Geometry: final body of the model. Coordinates: model frame, mm. A direction names the side the tool comes from. Give positions to 0.01 mm unless a question says otherwise; leave off trailing zeros. Loops run counter-clockwise (first coordinate to the right, second up) from the corner with the lowest first, then second, coordinate; pieces in that order, holes last. Notation, with made-up numbers: M 15.5,-31.75 L 69.5,-31.75 A20 ccw 69.5,-5.75 Z; hole C -32.5,-7 d9. An arc over 180 degrees is marked long. Put each result on its own line as item: value.
```python
from build123d import *

# Parameters (mm, degrees)
SKETCH2_W           = 22.4
SKETCH2_H           = 10
BOSS_EXTRUDE1_DEPTH = 14
CUT_EXTRUDE2_DEPTH  = 1.6
CUT_EXTRUDE4_DEPTH  = 13.4
BOSS_EXTRUDE2_DEPTH = 19
CUT_EXTRUDE5_DEPTH  = 27.105381484


with BuildPart() as part:
    # Sketch2 → Boss-Extrude1 (new body)
    with BuildSketch(Plane.XY):
        Rectangle(SKETCH2_W, SKETCH2_H)
    extrude(amount=BOSS_EXTRUDE1_DEPTH)

    # Sketch3 → Cut-Extrude2 (cut)
    with BuildSketch(Plane.XY.offset(14)):
        with BuildLine():
            Line((-6, 5), (6, 5))
            ThreePointArc((6, 5), (5.340169944, 2.204915028), (3.5, 0))
            Line((3.5, 0), (-3.5, 0))
            ThreePointArc((-3.5, 0), (-5.340169944, 2.204915028), (-6, 5))
        make_face()
    extrude(amount=-CUT_EXTRUDE2_DEPTH, mode=Mode.SUBTRACT)

    # Sketch5 → Cut-Extrude4 (cut, through all)
    with BuildSketch(Plane.XY.offset(12.4)):
        with BuildLine():
            Line((-6, 5), (6, 5))
            ThreePointArc((6, 5), (0, 2), (-6, 5))
        make_face()
    extrude(amount=-CUT_EXTRUDE4_DEPTH, mode=Mode.SUBTRACT)

    # Sketch6 → Boss-Extrude2 (add)
    with BuildSketch(Plane.XY):
        Polygon((-11.2, 5), (-13.2, 5), (-13.2, -7), (12.905381484, -7), (12.905381484, 5), (11.2, 5), (11.2, -5), (-11.2, -5), align=None)
    extrude(amount=BOSS_EXTRUDE2_DEPTH)

    # Sketch7 → Cut-Extrude5 (cut, through all)
    with BuildSketch(Plane.ZY.offset(13.2)):
        Polygon((0, 5), (14, 5), (0, 2), align=None)
    extrude(amount=-CUT_EXTRUDE5_DEPTH, mode=Mode.SUBTRACT)


solid = part.part
```
Item 1: Pin query (flat end, axial travel): pin 1 Ø1.4 at (x, y) = (-0.5, 2) entering from +Z; pin 2 Ø4 at (x, y) = (-7.5, -5.5) entering from -Z; pin 3 Ø1.8 at (x, z) = (-1.5, 13.5) entering from +Y; pin 4 Ø1 at (x, z) = (-9, 10.5) entering from +Y. Return the tip coordinate at first contact, or that it passes through.
Output values:
pin 1: z = 12.4
pin 2: z = 0
pin 3: y = 0
pin 4: y = 4.36
Item 2: Section A-A on y = 3.25. Output: boundary loops of the cut face in (x, z), then the cut area to 3 significant figures.
Output values:
outline: M -13.2,5.83 L -4.15,5.83 L -4.15,12.4 L -5.75,12.4 L -5.75,14 L -11.2,14 L -11.2,19 L -13.2,19 Z; M 4.15,5.83 L 12.91,5.83 L 12.91,19 L 11.2,19 L 11.2,14 L 5.75,14 L 5.75,12.4 L 4.15,12.4 Z
area: 159 mm²
Item 3: Mould query, pull axis X, two halves, no side actions, for faces 1 (the flat face through (12, 5, 16)), 2 (the flat face through (0, -5, 16)), 3 (the flat face through (-13.2, -1, 9)). Classes: pulls with the +X half, pulls with the -X half, needs draft (parallel to the pull), parting line crosses it, or undercut.
Output values:
face 1: needs draft
face 2: undercut
face 3: pulls with the -X half
Item 4: Section D-D on z = 13. Output: boundary loops of the cut face in (x, y), then the cut area to 3 significant figures.
Output values:
outline: M -13.2,-7 L 12.91,-7 L 12.91,4.79 L 6,4.79 A6.25 cw 3.5,0 L -3.5,0 A6.25 cw -6,4.79 L -13.2,4.79 Z
area: 258 mm²
Item 5: Section B-B on x = -11.5. Output: boundary loops of the cut face in (y, z).
Output values:
outline: M -7,0 L 2,0 L 5,14 L 5,19 L -7,19 Z
Item 6: Set-up query: faces 4 (the flat face through (0, -7, 9)), 5 (the cylindrical face through (5.358, 2.241, 13.211)). Return all of +Z, -Z, +X, -X, +Y, -Y with unobstructed straight access to the full face (end or side cutting, diameter ignored); none if empty.
Output values:
face 4: +Z, -Z, +X, -X, -Y
face 5: +Z, +Y
Item 7: Section C-C on y = -4. Output: boundary loops of the cut face in (x, z), then the cut area to 3 significant figures.
Output values:
outline: M -13.2,0 L 12.91,0 L 12.91,19 L 11.2,19 L 11.2,14 L -11.2,14 L -11.2,19 L -13.2,19 Z
area: 384 mm²
Item 8: Line query: probe 1 along X at (y, z) = (1, 15.5); probe 2 along Z at (x, y) = (-3.5, 1.75); probe 3 along Y at (x, z) = (5.75, 18). Output: solid intervals per line, ascending. Write a range as [from, to].
Output values:
probe 1: [-13.2, -11.2], [11.2, 12.91]
probe 2: [0, 12.4]
probe 3: [-7, -5]
